Autodesk Inventor part; units mm, degrees
ref_plane "YZ Plane" through (0, 0, 0) normal (1, 0, 0) x (0, 1, 0)
ref_plane "XZ Plane" through (0, 0, 0) normal (0, 1, 0) x (-1, 0, 0)
ref_plane "XY Plane" through (0, 0, 0) normal (0, 0, 1) x (1, 0, 0)
sketch "Sketch1" plane through (0, 0, 0) normal (0, 0, 1) x (1, 0, 0)
  line L0 (0, 0) -> (175, 0)
  line L1 (175, 0) -> (175, 75)
  line L2 (175, 75) -> (0, 75)
  line L3 (0, 75) -> (0, 0)
  dimension "d0" = 175
  dimension "d1" = 75
extrude "Extrusion1" add sketch "Sketch1" along normal blind 6.731
sketch "Sketch2" plane through (0, 0, 6.731) normal (0, 0, 1) x (1, 0, 0)
  line L0 (0, 0) -> (175, 0)
  line L1 (175, 0) -> (175, 75)
  line L2 (175, 75) -> (0, 75)
  line L3 (0, 75) -> (0, 0)
  line L4 (61.6333, 19.24) -> (144.1833, 19.24)
  line L5 (144.1833, 19.24) -> (144.1833, 67.5)
  line L6 (144.1833, 67.5) -> (137.8333, 67.5)
  line L7 (137.8333, 67.5) -> (62.9033, 67.5)
  line L8 (62.9033, 67.5) -> (61.6333, 67.5)
  line L9 (61.6333, 67.5) -> (61.6333, 19.24)
  dimension "d9" = 1.27
  dimension "d10" = 48.26
  dimension "d12" = 82.55
  dimension "d13" = 74.93
  dimension "d15" = 61.6333
  dimension "d16" = 30.8167
  dimension "d17" = 7.5
hole "Hole1" at (62.9033, 67.5, 6.731) at (144.1833, 19.24, 6.731) at (61.6333, 19.24, 6.731) at (137.8333, 67.5, 6.731) direction (0, 0, -1) diameter 3.176 end through all
sketch "Sketch3" plane through (0, 0, 6.731) normal (0, 0, 1) x (1, 0, 0)
  line L0 (0, 0) -> (175, 0)
  line L1 (175, 0) -> (175, 75)
  line L2 (0, 75) -> (0, 0)
  line L3 (72.5, 0) -> (102.5, 0)
  line L4 (102.5, 0) -> (102.5, -6.731)
  line L5 (102.5, -6.731) -> (72.5, -6.731)
  line L6 (72.5, -6.731) -> (72.5, 0)
  line L7 (0, 40) -> (-6.731, 40)
  line L8 (-6.731, 40) -> (-6.731, 20)
  line L9 (-6.731, 20) -> (0, 20)
  line L10 (0, 20) -> (0, 40)
  line L11 (175, 40) -> (181.731, 40)
  line L12 (181.731, 40) -> (181.731, 20)
  line L13 (181.731, 20) -> (175, 20)
  line L14 (175, 20) -> (175, 40)
  point P0 (87.5, -6.731)
  point P1 (87.5, 0)
  point P2 (-6.731, 30)
  point P3 (181.731, 30)
  dimension "d25" = 6.731
  dimension "d26" = 30
  dimension "d29" = 20
  dimension "d31" = 20
extrude "Extrusion2" add sketch "Sketch3" against normal blind 6.731
fillet "Fillet1" radius 2 2 edges at (0, 75, 3.3655) (175, 75, 3.3655)
equation "\"d7\" = THICKB"
equation "\"d15\" = 2 * d16"
equation "\"d25\" = THICKB"
equation "\"d27\" = THICKB"
equation "\"THICKA\" = 3.175"
equation "\"THICKB\" = 6.731"
equation "\"THICKC\" = 12.7"
equation "\"THICKPLY\" = 5"
equation "\"MAGDIA\" = 9.5"
equation "\"BALLDIA\" = 12"
properties part number "Mount_Mega_Bottom"
Build history of the part. All positions in model axes, mm. A direction names the side the tool comes from. Round coordinates to 2 decimals unless told otherwise and drop trailing zeros. Write each loop counter-clockwise with the first axis right and the second up, starting at its lowest first coordinate (ties: lowest second). Pieces come first, ordered by that corner, then holes. Notation, with made-up numbers: (-4.5, 22.25) - (22.5, 22.25) arc R31 ccw to (22.5, 55.25) - close; hole circle Ø10 at (71, 22.5). An arc over 180 degrees is marked (long way). One line per question, with ' | ' between items.
1. Band-saw the part on A-A, the plane z = 1.5. Write the cut outline in (x, y), and give its area (3 significant figures).
Results are:
outline: (-6.73, 20) - (0, 20) - (0, 0) - (72.5, 0) - (72.5, -6.73) - (102.5, -6.73) - (102.5, 0) - (175, 0) - (175, 20) - (181.73, 20) - (181.73, 40) - (175, 40) - (175, 73) arc R2 ccw to (173, 75) - (2, 75) arc R2 ccw to (0, 73) - (0, 40) - (-6.73, 40) - close; hole circle Ø3.18 at (61.63, 19.24); hole circle Ø3.18 at (62.9, 67.5); hole circle Ø3.18 at (137.83, 67.5); hole circle Ø3.18 at (144.18, 19.24) | area: 13,600 mm^2
2. Drop flat-ended pins along their axis: pin 1 Ø3.5 at (x, z) = (23, 3.5) entering from -Y; pin 2 Ø3.5 at (x, z) = (178, 2) entering from -Y. Give the stop position or say it passes through.
Results are:
pin 1: y = 0 | pin 2: y = 20
3. Band-saw the part on B-B, the plane x = 51.5. Write the cut outline in (y, z), and give its area (3 significant figures).
Results are:
outline: (0, 0) - (75, 0) - (75, 6.73) - (0, 6.73) - close | area: 505 mm^2
4. Tool access for faces 1 (the face through (36, 0, 3)), 2 (the face through (178, 20, 3)), 3 (the face through (-3, 40, 3)): list every direction of +Z, -Z, +X, -X, +Y, -Y with a clear straight run to the whole face (end or side of a thin tool).
Results are:
face 1: +Z, -Z, -X, -Y | face 2: +Z, -Z, +X, -Y | face 3: +Z, -Z, -X, +Y
5. Band-saw the part on C-C, the plane y = 9. Write the cut outline in (x, z).
Results are:
outline: (0, 0) - (175, 0) - (175, 6.73) - (0, 6.73) - close
6. Drill centre lines: line 1 along X through (y, z) = (19.24, 2); line 2 along X through (y, z) = (67.5, 3); line 3 along X through (y, z) = (13, 2.25). Where is each one in solid material? Low to high. Write a range as from..to.
Results are:
line 1: 0..60.05, 63.22..142.6, 145.77..175 | line 2: 0..61.32, 64.49..136.25, 139.42..175 | line 3: 0..175
7. Mould opens along X. For faces 4 (the face through (0, 10, 3)), 5 (the face through (102.5, -3, 3)), 6 (the face through (60.06, 19.45, 3.32)), 7 (the face through (142.61, 19.45, 3.32)) say: released by +X, released by -X, zero draft, split by the parting line, or undercut.
Results are:
face 4: released by -X | face 5: released by +X | face 6: undercut | face 7: undercut
